Input: dimensioned drawing with shaded views. Units: mm. Origin: part minimum x, y, z. A direction names the side the tool comes from. Give positions to 0.01 mm unless a question says otherwise; leave off trailing zeros. Write each loop counter-clockwise with the first axis right and the second up, starting at its lowest first coordinate (ties: lowest second). Pieces come first, ordered by that corner, then holes.
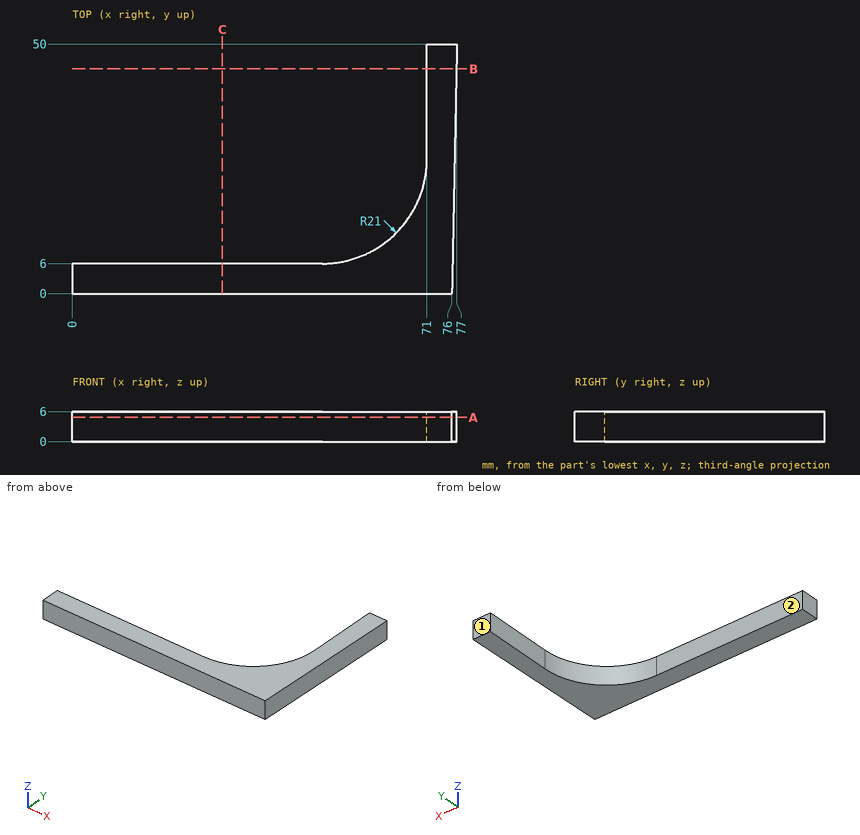
Item 1: Section A-A, the plane z = 4.85. Return the cut outline in (x, y).
Found:
outline: (0, 0) - (76, 0) - (77, 50) - (71, 50) - (71, 27) arc R21 cw to (50, 6) - (0, 6) - close
Item 2: Line query: L1, parallel to Y at x = 36, z = 1.55; L2, parallel to X at y = 34, z = 0.45; L3, parallel to Y at x = 61, z = 4.1. Output: solid intervals per line, ascending.
Found:
L1: y = 0 to 6
L2: x = 71 to 76.68
L3: y = 0 to 9.11
Item 3: Section C-C, the plane x = 30. Return the cut outline in (y, z).
Found:
outline: (0, 0) - (6, 0) - (6, 6) - (0, 6) - close
Item 4: Pin query (flat end, axial travel): pin 1 Ø2 at (x, z) = (56, 4) entering from +Y; pin 2 Ø1.5 at (x, z) = (19, 2) entering from +Y. Return the tip coordinate at first contact, or that it passes through.
Found:
pin 1: stops at y = 7.2
pin 2: stops at y = 6
Item 5: Reachability of the marked faces 1 and 2 from +Z, -Z, +X, -X, +Y, -Y: full face, straight path, thin tool, end or side. Return the list, or none.
Found:
face 1: +Z, -Z, +X, -X, +Y
face 2: +Z, -Z, -X, +Y
Item 6: Section B-B, the plane y = 45. Return the cut outline in (x, z), plus the area to 3 significant figures.
Found:
outline: (71, 0) - (76.9, 0) - (76.9, 6) - (71, 6) - close
area: 35.4 mm2
